Input: part model. Units: mm. Frame: model coordinates. Face numbers are marked on the shaded views. A direction names the side the tool comes from. Coordinates: 2 decimals unless noted, no trailing zeros. Order: outer loops, then holes, each group sorted by start corner. A loop starts at its lowest first (then second) coordinate and runs counter-clockwise, first axis right, second up.
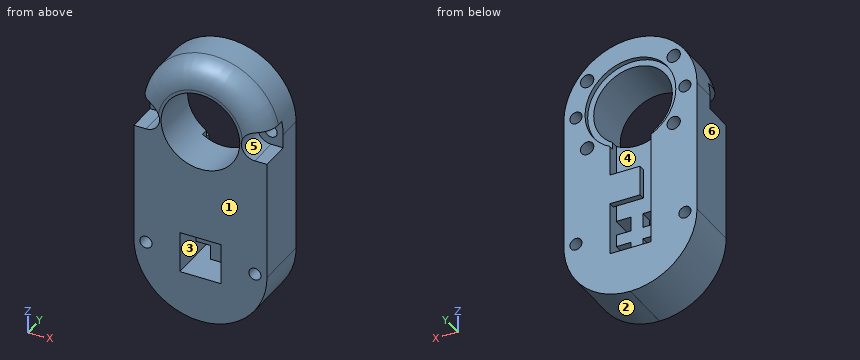
from build123d import *

# Parameters (mm, degrees)
SKETCH1_R           = 6.5
BOSS_EXTRUDE1_DEPTH = 9
SKETCH2_R           = 1.1
CUT_EXTRUDE1_DEPTH  = 3
SKETCH3_R           = 1
CUT_EXTRUDE2_DEPTH  = 20
CUT_EXTRUDE3_DEPTH  = 5
SKETCH6_W           = 6.8
SKETCH6_H           = 6.8
CUT_EXTRUDE4_DEPTH  = 5
SKETCH7_W           = 2.4
SKETCH7_H           = 2.4
CUT_EXTRUDE5_DEPTH  = 5
FILLET2_R           = 4
SKETCH8_R           = 1
CUT_EXTRUDE6_DEPTH  = 20
SKETCH9_R           = 7.5
CUT_EXTRUDE7_DEPTH  = 0.8
SKETCH10_W          = 6.8
SKETCH10_H          = 19.870144406
CUT_EXTRUDE8_DEPTH  = 2
SKETCH11_W          = 5
SKETCH11_H          = 1
BOSS_EXTRUDE2_DEPTH = 5


with BuildPart() as part:
    # Sketch1 → Boss-Extrude1 (new body)
    with BuildSketch(Plane(origin=(0, 0, 0), x_dir=(1, 0, 0), z_dir=(0, 1, 0))):
        with BuildLine():
            Line((-11, 0), (-11, 22.01))
            ThreePointArc((-11, 22.01), (-7.781103525, 29.781103525), (-0.01, 33))
            Line((-0.01, 33), (0.01, 33))
            ThreePointArc((0.01, 33), (7.781103525, 29.781103525), (11, 22.01))
            Line((11, 22.01), (11, 0))
            ThreePointArc((11, 0), (0, -11), (-11, 0))
        make_face()
        Circle(SKETCH1_R, mode=Mode.SUBTRACT)
    extrude(amount=BOSS_EXTRUDE1_DEPTH)

    # Sketch2 → Cut-Extrude1 (cut)
    with BuildSketch(Plane(origin=(0, 9, 0), x_dir=(1, 0, 0), z_dir=(0, 1, 0))):
        with Locations((-7.15, 5.85)):
            Circle(SKETCH2_R)
        with Locations((-7.15, -5.85)):
            Circle(SKETCH2_R)
        with Locations((7.15, -5.85)):
            Circle(SKETCH2_R)
        with Locations((7.15, 5.85)):
            Circle(SKETCH2_R)
    extrude(amount=-CUT_EXTRUDE1_DEPTH, mode=Mode.SUBTRACT)

    # Sketch3 → Cut-Extrude2 (cut)
    with BuildSketch(Plane(origin=(0, 9, 0), x_dir=(1, 0, 0), z_dir=(0, 1, 0))):
        with Locations((-9, 0)):
            Circle(SKETCH3_R)
        with Locations((9, 0)):
            Circle(SKETCH3_R)
    extrude(amount=-CUT_EXTRUDE2_DEPTH, mode=Mode.SUBTRACT)

    # Sketch4 → Cut-Extrude3 (cut)
    with BuildSketch(Plane.XZ):
        with BuildLine():
            Line((-9, 2.25), (-10.767427734, 2.25))
            Line((-10.767427734, 2.25), (-12, 0))
            Line((-12, 0), (-11, -2.25))
            Line((-11, -2.25), (-9, -2.25))
            ThreePointArc((-9, -2.25), (-6.75, 0), (-9, 2.25))
        make_face()
        with BuildLine():
            Line((12, 0), (10.767427734, 2.25))
            Line((10.767427734, 2.25), (9, 2.25))
            ThreePointArc((9, 2.25), (6.75, 0), (9, -2.25))
            Line((9, -2.25), (11, -2.25))
            Line((11, -2.25), (12, 0))
        make_face()
    extrude(amount=-CUT_EXTRUDE3_DEPTH, mode=Mode.SUBTRACT)

    # Sketch6 → Cut-Extrude4 (cut)
    with BuildSketch(Plane.XZ):
        with Locations((0, -22.01)):
            Rectangle(SKETCH6_W, SKETCH6_H)
    extrude(amount=-CUT_EXTRUDE4_DEPTH, mode=Mode.SUBTRACT)

    # Sketch7 → Cut-Extrude5 (cut)
    with BuildSketch(Plane.XZ.offset(-5)):
        with Locations((2.2, -19.81)):
            Rectangle(SKETCH7_W, SKETCH7_H)
        with Locations((-2.2, -19.81)):
            Rectangle(SKETCH7_W, SKETCH7_H)
        with Locations((2.2, -24.21)):
            Rectangle(SKETCH7_W, SKETCH7_H)
        with Locations((-2.2, -24.21)):
            Rectangle(SKETCH7_W, SKETCH7_H)
    extrude(amount=-CUT_EXTRUDE5_DEPTH, mode=Mode.SUBTRACT)

    # Fillet2
    fillet2_edges = [part.edges().sort_by_distance(p)[0] for p in [
        (0, 0, 11),
    ]]
    fillet(fillet2_edges, radius=FILLET2_R)

    # Sketch8 → Cut-Extrude6 (cut)
    with BuildSketch(Plane.XZ):
        with Locations((-9, -22.01)):
            Circle(SKETCH8_R)
        with Locations((9, -22.01)):
            Circle(SKETCH8_R)
    extrude(amount=-CUT_EXTRUDE6_DEPTH, mode=Mode.SUBTRACT)

    # Sketch9 → Cut-Extrude7 (cut)
    with BuildSketch(Plane(origin=(0, 9, 0), x_dir=(1, 0, 0), z_dir=(0, 1, 0))):
        Circle(SKETCH9_R)
    extrude(amount=-CUT_EXTRUDE7_DEPTH, mode=Mode.SUBTRACT)

    # Sketch10 → Cut-Extrude8 (cut)
    with BuildSketch(Plane(origin=(0, 9, 0), x_dir=(1, 0, 0), z_dir=(0, 1, 0))):
        with Locations((0, 15.474927797)):
            Rectangle(SKETCH10_W, SKETCH10_H)
    extrude(amount=-CUT_EXTRUDE8_DEPTH, mode=Mode.SUBTRACT)

    # Sketch11 → Boss-Extrude2 (add)
    with BuildSketch(Plane.ZY.offset(-3.4)):
        with Locations((-14.185057965, 8.5)):
            Rectangle(SKETCH11_W, SKETCH11_H)
    extrude(amount=BOSS_EXTRUDE2_DEPTH)


solid = part.part
Item 1: Cut plane D-D on z = -28.5. Return loops of the section in (x, y).
Response values:
outline: (-8.88, 0) - (8.88, 0) - (8.88, 9) - (-8.88, 9) - close
Item 2: Access query for the marked faces 4, 5 and 6. Directions: +Z, -Z, +X, -X, +Y, -Y. A direction counts if a zero-diameter tool reaches every point of the face in a straight line with its end or side. Return the directions, or none.
Response values:
face 4: none
face 5: +X, -Y
face 6: +Z, -Z, -X, +Y, -Y
Item 3: Cut plane B-B on z = -10.5. Return loops of the section in (x, y).
Response values:
outline: (-11, 0) - (11, 0) - (11, 9) - (3.4, 9) - (3.4, 7) - (-3.4, 7) - (-3.4, 9) - (-11, 9) - close
Item 4: Draft query along X for the marked faces 1, 2 and 3. Return one class per face: pulls with the +X half, pulls with the -X half, needs draft (parallel to the pull), parting line crosses it, or undercut.
Response values:
face 1: needs draft
face 2: pulls with the +X half
face 3: undercut
Item 5: Cut plane C-C on x = -2.25. Count the separate pieces of the cut face and the enclosed holes in it, then the cut area to 3 significant figures.
Response values:
separate pieces: 4
enclosed holes: 0
area: 195 mm2
Item 6: Cut plane A-A on z = -19.5. Return loops of the section in (x, y), then the cut area to 3 significant figures.
Response values:
outline: (-11, 0) - (-3.4, 0) - (-3.4, 9) - (-11, 9) - close; (-1, 5) - (1, 5) - (1, 7) - (-1, 7) - close; (3.4, 0) - (11, 0) - (11, 9) - (3.4, 9) - close
area: 141 mm2
Item 7: Pin query (flat end, axial travel): pin 1 Ø3 at (x, z) = (-4, -21.5) entering from -Y; pin 2 Ø1.3 at (x, z) = (9.5, -1) entering from -Y; pin 3 Ø1 at (x, y) = (1.5, 6) entering from -Z; pin 4 Ø1.4 at (x, y) = (10, 2.5) entering from -Z. Return the tip coordinate at first contact, or that it passes through.
Response values:
pin 1: stops at y = 0
pin 2: stops at y = 5
pin 3: stops at z = -32.96
pin 4: stops at z = -27.88
Item 8: Ray query, probe 1 along X at (y, z) = (7.6, -5.85); probe 2 along Z at (x, y) = (-7.5, 6.5); probe 3 along X at (y, z) = (6.7, -5.85). Return the intervals inside material, ascending.
Response values:
probe 1: x = -11 to -8.25, -6.05 to -3.4, 3.4 to 6.05, 8.25 to 11
probe 2: z = -30.05 to -6.89, -4.81 to 4.81, 6.89 to 8.05
probe 3: x = -11 to -8.25, -6.05 to -2.83, 2.83 to 6.05, 8.25 to 11
